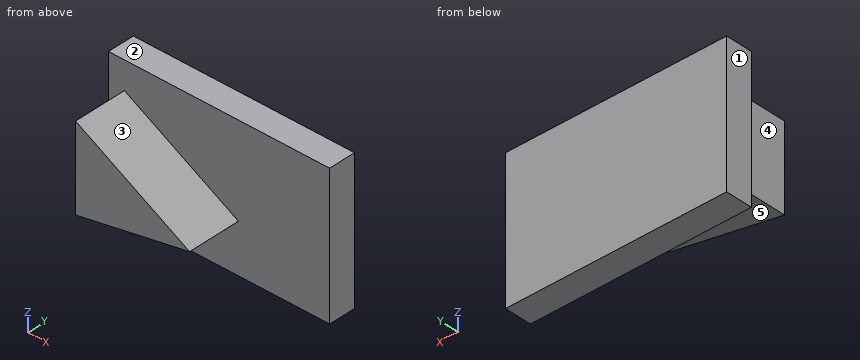
```python
from build123d import *

# Parameters (mm, degrees)
F0_W     = 208.097614
F0_H     = 131.79294
F1_DEPTH = 25.4
F4_DEPTH = 50


with BuildPart() as f1:
    # F0 (on Front) → F1 (new body)
    with BuildSketch(Plane.XZ):
        with Locations((-18.191915, 3.902476)):
            Rectangle(F0_W, F0_H)
    extrude(amount=F1_DEPTH)

    # F3 (on face) → F4 (join)
    with BuildSketch(Plane.XZ.offset(25.4)):
        Polygon((-107.326537, -35.649035), (0, -15.753135), (-107.326537, 43.823242), align=None)
    extrude(amount=F4_DEPTH)


solid = f1.part
```
CAD build for the part. Positions are in the model's coordinates, mm. Face numbers are marked on the shaded views. A direction names the side the tool comes from. Coordinates: 2 decimals unless noted, no trailing zeros. Write each loop counter-clockwise with the first axis right and the second up, starting at its lowest first coordinate (ties: lowest second). Pieces come first, ordered by that corner, then holes. Notation, with made-up numbers: (15.25, 52.5) -> (25.25, 52.5) arc R10 ccw to (25.25, 71.5) -> close; hole circle Ø9 at (-17.75, 11.5). An arc over 180 degrees is marked (long way). Return JSON: item names as keys, results as strings. Group by question number.
Q1. Cut at B-B, the plane z = 5.5. Give the cut face in (x, y).
Q2. Drill centre lines: line 1 (Y direction, x = -4.5, z = 48.5); line 2 (X direction, y = -48.5, z = 35.5); line 3 (Z direction, x = -100, y = -68.5). Where is each one in solid material? Low to high.
Q3. Cut at A-A, the plane x = -57.5. Give the cut face in (y, z).
Q4. Cut at D-D, the plane z = -45. Give the cut face in (x, y), then the cut area to 3 significant figures.
Q5. Cut at C-C, the plane y = -60. Give the cut face in (x, z).
Q6. Which spindle directions (+Z, -Z, +X, -X, +Y, -Y) get a long thin tool onto all of the face, cutting with end or side? Do the marked faces 1, 2, 3, 4 and 5. Say none if no direction does.
Q7. Flat gauge pins, fed straight in: pin 1 (10 mm diameter, centred on x = -96.5, y = -39.5, fed in from -Z); pin 2 (1 mm diameter, centred on x = -3.5, y = -67, fed in from -Z); pin 3 (25 mm diameter, centred on y = -49, z = -14, fed in from -X). Where does each tip first touch, or does it go through?
Returned:
{
 "1": {"outline": "(-122.24, -25.4) -> (-107.33, -25.4) -> (-107.33, -75.4) -> (-38.29, -75.4) -> (-38.29, -25.4) -> (85.86, -25.4) -> (85.86, 0) -> (-122.24, 0) -> close"},
 "2": {"line 1": "y = -25.4 to 0", "line 2": "x = -107.33 to -92.33", "line 3": "z = -34.29 to 39.76"},
 "3": {"outline": "(-75.4, -26.41) -> (-25.4, -26.41) -> (-25.4, -61.99) -> (0, -61.99) -> (0, 69.8) -> (-25.4, 69.8) -> (-25.4, 16.16) -> (-75.4, 16.16) -> close"},
 "4": {"outline": "(-122.24, -25.4) -> (85.86, -25.4) -> (85.86, 0) -> (-122.24, 0) -> close", "area": "5,290 mm2"},
 "5": {"outline": "(-107.33, -35.65) -> (0, -15.75) -> (-107.33, 43.82) -> close"},
 "6": {"face 1": "+Z, -Z, -X, +Y, -Y", "face 2": "+Z, +X, -X, +Y, -Y", "face 3": "+Z, +X, -Y", "face 4": "+Z, -Z, -X, -Y", "face 5": "-Z, +X, -Y"},
 "7": {"pin 1": "stops at z = -34.57", "pin 2": "stops at z = -16.49", "pin 3": "stops at x = -107.33"}
}
